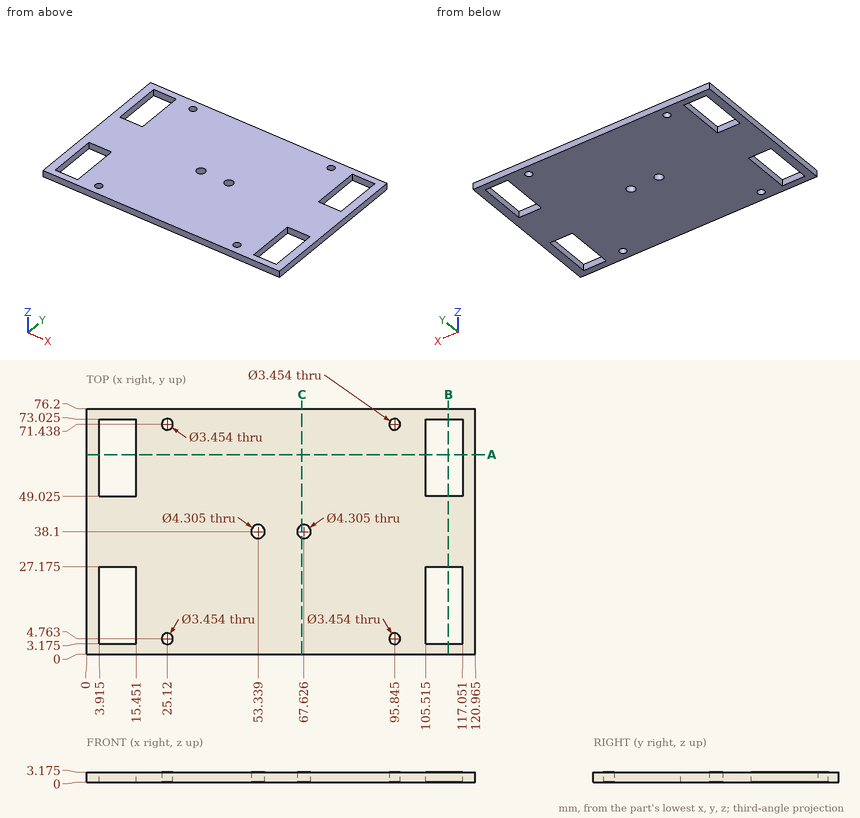
Answer from the drawing. Dimensions are ordinates in mm from the lowest x, y and z of the part. Give positions to 0.01 mm unless a question says otherwise; leave off trailing zeros. Loops run counter-clockwise (first coordinate to the right, second up) from the corner with the lowest first, then second, coordinate; pieces in that order, holes last. Notation, with made-up numbers: (-27.5, -6) - (-16.5, -6) arc R33 cw to (-16.5, 24) - close; hole circle Ø5 at (-8, 2.5). An arc over 180 degrees is marked (long way). Answer as a JSON object with one key per item and string values.
1. A flat-ended cylindrical pin translates along its axis: pin 1 Ø4 at (x, y) = (53.34, 38.1) entering from -Z. Find the tip coordinate at first contact, or state that the pin passes through.
Determined:
{"pin 1": "through"}
2. Find the intervals of material crossed by L1, parallel to Y at x = 110.5, z = 1.05 (1 decimal); L2, parallel to Y at x = 67, z = 2.25, in increasing order. Write a range as [from, to].
Determined:
{"L1": "[0, 3.2], [27.2, 49], [73, 76.2]", "L2": "[0, 36.04], [40.16, 76.2]"}
3. A cutting plane is placed at C-C (x = 67). Write down the section's boundary in (y, z) (1 decimal).
Determined:
{"outline": "(0, 0) - (36, 0) - (36, 3.2) - (0, 3.2) - close; (40.2, 0) - (76.2, 0) - (76.2, 3.2) - (40.2, 3.2) - close"}
4. A cutting plane is placed at B-B (x = 112.5). Write down the section's boundary in (y, z) (1 decimal).
Determined:
{"outline": "(0, 0) - (3.2, 0) - (3.2, 3.2) - (0, 3.2) - close; (27.2, 0) - (49, 0) - (49, 3.2) - (27.2, 3.2) - close; (73, 0) - (76.2, 0) - (76.2, 3.2) - (73, 3.2) - close"}
5. A cutting plane is placed at A-A (y = 62). Give the number of separate pieces and of enclosed holes in the cut face, then the cut area to 3 significant figures.
Determined:
{"separate pieces": "3", "enclosed holes": "0", "area": "311 mm²"}
